from build123d import *


with BuildPart() as f1:
    # F0 (on Front) → F1 (revolve)
    with BuildSketch(Plane.XZ):
        with BuildLine():
            Line((-101.6, 0), (0, 0))
            Line((0, 0), (0, 19.05))
            ThreePointArc((0, 19.05), (-1.859872, 23.540128), (-6.35, 25.4))
            Line((-6.35, 25.4), (-82.55, 25.4))
            ThreePointArc((-82.55, 25.4), (-87.040128, 23.540128), (-88.9, 19.05))
            ThreePointArc((-88.9, 19.05), (-90.759872, 14.559872), (-95.25, 12.7))
            Line((-95.25, 12.7), (-101.6, 12.7))
            Line((-101.6, 12.7), (-101.6, 0))
        make_face()
    revolve(axis=Axis((-50.8, 0, 0), (-1, 0, 0)))


solid = f1.part
Build history of the part. All positions in model axes, mm. A direction names the side the tool comes from. Coordinates: 2 decimals unless noted, no trailing zeros. Order: outer loops, then holes, each group sorted by start corner. A loop starts at its lowest first (then second) coordinate and runs counter-clockwise, first axis right, second up. Notation, with made-up numbers: (-20, 23) -> (-15, 23) arc R13 cw to (-15, 39) -> close; hole circle Ø9 at (-22.75, 8). An arc over 180 degrees is marked (long way). One line per item, written item: value.
(1) Slice it at A-A, the plane x = -46. List the corners of the cut face in (y, z), plus the area to 3 significant figures.
Checked values:
outline: circle Ø50.8 at (0, 0)
area: 2,030 mm2
(2) Tool access for faces 1 (the cylindrical face through (-98.47, -12.4, -2.75)), 2 (the flat face through (-101.6, 0, 0)): list every direction of +Z, -Z, +X, -X, +Y, -Y with a clear straight run to the whole face (end or side of a thin tool).
Checked values:
face 1: -X
face 2: +Z, -Z, -X, +Y, -Y
(3) Probe line 1 (X direction, y = -9, z = -17); line 2 (Y direction, x = -50, z = -0.5); line 3 (Z direction, x = -39, y = 7). List the from-to ranges inside material, lowest first. Write a range as [from, to].
Checked values:
line 1: [-88.9, 0]
line 2: [-25.4, 25.4]
line 3: [-24.42, 24.42]
(4) Drop flat-ended pins along their axis: pin 1 Ø1 at (x, y) = (-41.5, 18.5) entering from +Z; pin 2 Ø1.5 at (x, y) = (-14.5, 10.5) entering from +Z; pin 3 Ø3 at (x, y) = (-16, 15) entering from -Z. Give the stop position or say it passes through.
Checked values:
pin 1: z = 17.92
pin 2: z = 23.45
pin 3: z = -21.52
